Here's the drawing with two shaded views (mm, measured from the low corner). I have some questions. A direction names the side the tool comes from. Coordinates: 2 decimals unless noted, no trailing zeros. Write each loop counter-clockwise with the first axis right and the second up, starting at its lowest first coordinate (ties: lowest second). Pieces come first, ordered by that corner, then holes. Notation, with made-up numbers: M -39,46.5 L 1,46.5 A27 cw 1,82.5 Z; hole C 5.5,24.5 d9. An arc over 180 degrees is marked long. Answer as CSV lines item,"result". Start each with the question number.
Item 1: Suppose I cut it at B-B, the plane x = 5. Write out the boundary of the cut face in (y, z), and give its area (3 significant figures).
Item 2: If I drill on line 1 along Y through (x, z) = (3.9, 5); line 2 along Y through (x, z) = (1.5, 5); line 3 along X through (y, z) = (4.25, 5), over which ranges is the centre line in solid material (lowest first)? Write a range as [from, to].
Item 3: Suppose I cut it at C-C, the plane y = 21.75. Write out the boundary of the cut face in (x, z), and give its area (3 significant figures).
Item 4: Suppose I cut it at D-D, the plane z = 3. Write out the boundary of the cut face in (x, y).
Item 5: Suppose I cut it at A-A, the plane z = 5. Write out the boundary of the cut face in (x, y).
Item 6: We'd pull the mould along Y, two halves only. Please class the marked faces 3, 4, 5 and 6: +Y half, -Y half, draft (parallel to the pull), parting line (faces both ways), or undercut.
Item 7: On a 3-axis mill with a long thin cutter (end or side, diameter ignored), from which of +Z, -Z, +X, -X, +Y, -Y can I reach the whole of each face in a straight line? I mean the marked faces 1 and 2. Say none if no direction works.
Item 8: I'm going to push flat-ended pins straight in: P1, Ø3, axis at y = 2, z = 5, coming from the -X side; P2, Ø6, axis at y = 17.5, z = 2, coming from the +X side; P3, Ø3, axis at y = 20.5, z = 8, coming from the -X side. Where does each tip first touch, or does it pass through?
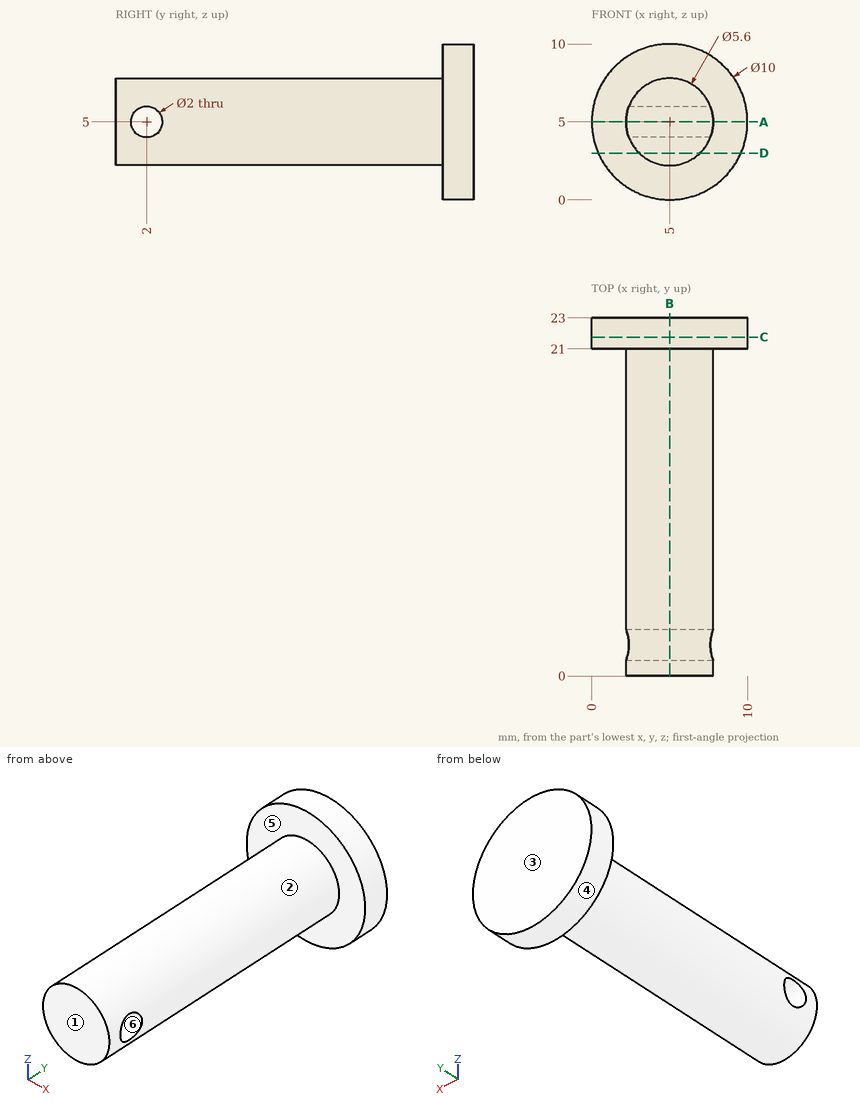
Ans:
1,outline,"M 0,2.2 L 21,2.2 L 21,0 L 23,0 L 23,10 L 21,10 L 21,7.8 L 0,7.8 Z; hole C 2,5 d2"
1,area,"134 mm^2"
2,line 1,"y = [0, 1], [3, 23]"
2,line 2,"y = [21, 23]"
2,line 3,"x = [2.2, 7.8]"
3,outline,"C 5,5 d10"
3,area,"78.5 mm^2"
4,outline,"M 0.42,21 L 3.04,21 L 3.04,0 L 6.96,0 L 6.96,21 L 9.58,21 L 9.58,23 L 0.42,23 Z"
5,outline,"M 0,21 L 2.2,21 L 2.2,3 L 7.8,3 L 7.8,21 L 10,21 L 10,23 L 0,23 Z; M 2.2,0 L 7.8,0 L 7.8,1 L 2.2,1 Z"
6,face 3,"+Y half"
6,face 4,"draft"
6,face 5,"-Y half"
6,face 6,"undercut"
7,face 1,"+Z, -Z, +X, -X, -Y"
7,face 2,"-Y"
8,P1,"stops at x = 2.2"
8,P2,"stops at x = 7.8"
8,P3,"stops at x = 0.26"
